Study the drawing (mm; zero at the part's minimum x, y, z) and answer. A direction names the side the tool comes from. Give positions to 0.01 mm unless a question says otherwise; leave off trailing zeros. Loops run counter-clockwise (first coordinate to the right, second up) from the corner with the lowest first, then second, coordinate; pieces in that order, holes last. Notation, with made-up numbers: M 83.5,30.25 L 95.5,30.25 A11 ccw 95.5,39.25 Z; hole C 33,60.25 d4. An arc over 180 degrees is marked long. Use one line per item in the form item = value. Start each with the question number.
1. The part is cut by section C-C (z = 52). Write down the section's boundary in (x, y), and give its area (3 significant figures).
2. Each of these flat-tipped pins is pushed along its axis until it touches: pin 1 Ø1 at (x, y) = (44.5, 3.5) entering from -Z; pin 2 Ø6 at (x, z) = (40, 33) entering from -Y; pin 3 Ø2 at (x, z) = (50, 41) entering from -Y; pin 4 Ø1.3 at (x, z) = (31, 53) entering from +Y. Where does it stop, or does it pass through?
3. The part is cut by section A-A (x = 20). Write down the section's boundary in (y, z).
4. The part is cut by section B-B (y = 18.5). Write down the section's boundary in (x, z), and give its area (3 significant figures).
5. Straight lines are drawn through the part: line 1 (X direction, y = 18.25, z = 52); line 2 (Z direction, x = 19.5, y = 21.5); line 3 (Z direction, x = 40, y = 5.5). For each, find the intervals that lie inside material, in ascending order. Write a range as from..to.
6. The mould has two halves that part along Z. Classify the marked faces 1, 2 and 3: released by +Z, released by -Z, zero draft, split by the parting line, or undercut.
7. For the marked faces 4 and 5, determine the directions among +Z, -Z, +X, -X, +Y, -Y from which every point of the face is accessible in a straight line to the end or side of a thin tool.
8. The part is cut by section D-D (z = 26). Write down the section's boundary in (x, y).
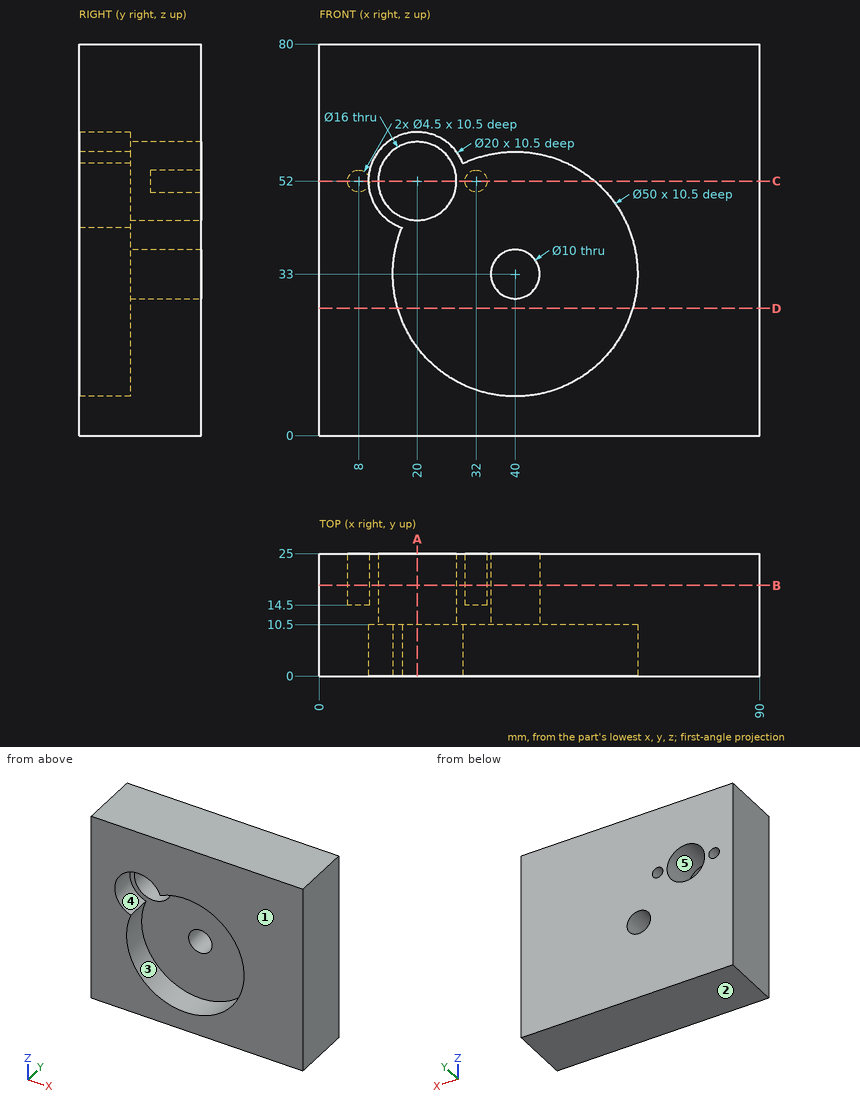
Derived:
q1.outline = M 0,0 L 10,0 L 10,10.5 L 12,10.5 L 12,25 L 10.25,25 L 10.25,14.5 L 5.75,14.5 L 5.75,25 L 0,25 Z; M 28,10.5 L 56.25,10.5 L 56.25,0 L 90,0 L 90,25 L 34.25,25 L 34.25,14.5 L 29.75,14.5 L 29.75,25 L 28,25 Z
q1.area = 1,440 mm2
q2.pin_1 = 0
q2.pin_2 = through
q2.pin_3 = 10.5
q2.pin_4 = 14.5
q3.outline = M 0,0 L 25,0 L 25,44 L 10.5,44 L 10.5,18 L 0,18 Z; M 0,62 L 10.5,62 L 10.5,60 L 25,60 L 25,80 L 0,80 Z
q4.outline = M 0,0 L 90,0 L 90,80 L 0,80 Z; hole C 8,52 d4.5; hole C 20,52 d16; hole C 32,52 d4.5; hole C 40,33 d10
q4.area = 6,890 mm2
q5.line_1 = 0..5.75, 10.25..12, 28..29.75, 34.25..90
q5.line_2 = 0..44.02, 59.98..80
q5.line_3 = 0..8, 58..80
q6.face_1 = zero draft
q6.face_2 = released by -Z
q6.face_3 = undercut
q7.face_4 = -Y
q7.face_5 = +Y, -Y
q8.outline = M 0,0 L 16,0 L 16,10.5 L 64,10.5 L 64,0 L 90,0 L 90,25 L 0,25 Z
